```python
from build123d import *

# Parameters (mm, degrees)
SKETCH1_W               = 27
SKETCH1_H               = 22
SKETCH1_R               = 1.5
BOSS_EXTRUDE1_DEPTH     = 3
SKETCH2_W               = 3.5
SKETCH2_H               = 17
BOSS_EXTRUDE2_DEPTH     = 17
CUT_EXTRUDE1_DEPTH      = 28.451092874
CUT_EXTRUDE1_DEPTH_BACK = 28.451092874
SKETCH3_R               = 4
CUT_EXTRUDE2_DEPTH      = 28.451092874
CUT_EXTRUDE2_DEPTH_BACK = 28.451092874
SKETCH4_W               = 8.09758535
SKETCH4_H               = 1.5
FILLET1_R               = 3
FILLET2_R               = 3


with BuildPart() as part:
    # Sketch1 → Boss-Extrude1 (new body)
    with BuildSketch(Plane.XY):
        Rectangle(SKETCH1_W, SKETCH1_H)
        with Locations((10.5, 8.5)):
            Circle(SKETCH1_R, mode=Mode.SUBTRACT)
        with Locations((10.5, -8.5)):
            Circle(SKETCH1_R, mode=Mode.SUBTRACT)
        with Locations((-10.5, -8.5)):
            Circle(SKETCH1_R, mode=Mode.SUBTRACT)
        with Locations((-10.5, 8.5)):
            Circle(SKETCH1_R, mode=Mode.SUBTRACT)
    extrude(amount=BOSS_EXTRUDE1_DEPTH)

    # Sketch2 → Boss-Extrude2 (add)
    with BuildSketch(Plane.XY.offset(3)):
        Rectangle(SKETCH2_W, SKETCH2_H)
    extrude(amount=BOSS_EXTRUDE2_DEPTH)

    # Sketch3 → Cut-Extrude1 (cut, two sides: drawn at the far end of the back side and taken through both)
    with BuildSketch(Plane(origin=(1.75, 0, 0), x_dir=(0, 0, -1), z_dir=(1, 0, 0)).offset(-CUT_EXTRUDE1_DEPTH_BACK)):
        with Locations(Location((-13, 0, 0), (0, 0, 90))):
            Circle(SKETCH3_R)
    extrude(amount=CUT_EXTRUDE1_DEPTH + CUT_EXTRUDE1_DEPTH_BACK, mode=Mode.SUBTRACT)

    # Sketch4 → Cut-Extrude2 (cut, two sides: drawn at the far end of the back side and taken through both)
    with BuildSketch(Plane(origin=(1.75, 0, 0), x_dir=(0, 0, -1), z_dir=(1, 0, 0)).offset(-CUT_EXTRUDE2_DEPTH_BACK)):
        with Locations((-18.330812417, 0)):
            Rectangle(SKETCH4_W, SKETCH4_H)
    extrude(amount=CUT_EXTRUDE2_DEPTH + CUT_EXTRUDE2_DEPTH_BACK, mode=Mode.SUBTRACT)

    # Fillet1
    fillet1_edges = [part.edges().sort_by_distance(p)[0] for p in [
        (-1.75, 0, 3),
        (1.75, 0, 3),
    ]]
    fillet(fillet1_edges, radius=FILLET1_R)

    # Fillet2
    fillet2_edges = [part.edges().sort_by_distance(p)[0] for p in [
        (0, -8.5, 20),
        (0, 8.5, 20),
    ]]
    fillet(fillet2_edges, radius=FILLET2_R)


solid = part.part
```
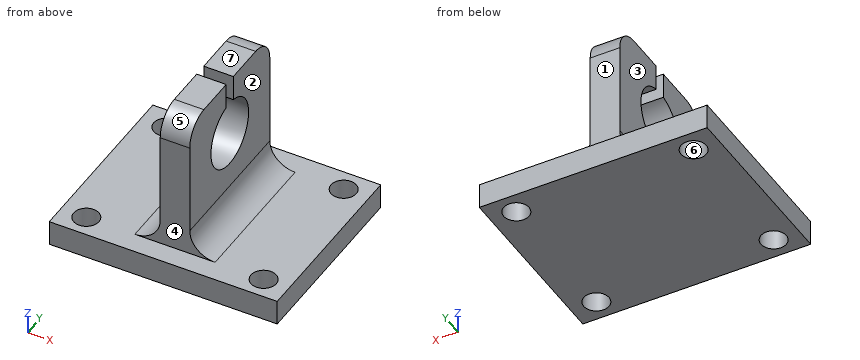
Could you check a few things on this model? Use its own coordinates, in mm. Face numbers are marked on the shaded views. A direction names the side the tool comes from. Round coordinates to 2 decimals unless told otherwise and drop trailing zeros. Loops run counter-clockwise (first coordinate to the right, second up) from the corner with the lowest first, then second, coordinate; pieces in that order, holes last. Notation, with made-up numbers: M 53.5,53 L 103.5,53 A35 ccw 103.5,91 Z; hole C 64.25,68.5 d9. An arc over 180 degrees is marked long. Write item = value, one per line.
1. Which directions (+Z, -Z, +X, -X, +Y, -Y) give clear straight access to the entire face, cutting with the end or side of a thin tool? Please do the marked faces 1, 2, 3 and 4.
Results below:
face_1 = +Z, +X, -X, +Y
face_2 = +Z, +X, +Y, -Y
face_3 = +Z, -X, +Y, -Y
face_4 = +Z, +X, -X, -Y
2. Will these pins go through, and if not, where does the flat tip stop? P1, Ø7, axis at y = 0, z = 13, coming from the -X side; P2, Ø7, axis at y = -1.5, z = 11.5, coming from the +X side; P3, Ø10, axis at x = -9.5, y = 5, coming from the +Z side; P4, Ø3, axis at x = -1.5, z = 9.5, coming from the +Y side.
Results below:
P1 = through
P2 = 1.75
P3 = 3.01
P4 = 8.5
3. I want a section at D-D, the plane y = 9. Write out the boundary of the cut face in (x, z), and give its area (3 significant figures).
Results below:
outline = M -13.5,0 L -11.91,0 L -11.91,3 L -13.5,3 Z; M -9.09,0 L 9.09,0 L 9.09,3 L -9.09,3 Z; M 11.91,0 L 13.5,0 L 13.5,3 L 11.91,3 Z
area = 64.0 mm²
4. I want a section at C-C, the plane y = 0. Write out the boundary of the cut face in (x, z), and give its area (3 significant figures).
Results below:
outline = M -13.5,0 L 13.5,0 L 13.5,3 L 4.75,3 A3 cw 1.75,6 L 1.75,9 L -1.75,9 L -1.75,6 A3 cw -4.75,3 L -13.5,3 Z
area = 106 mm²
5. Thinking about a two-plate mould opening in Y: for the marked faces 5, 6 and 7, which applies, +Y half, -Y half, draft (parallel to the pull), parting line (faces both ways), or undercut?
Results below:
face_5 = -Y half
face_6 = undercut
face_7 = draft
6. I want a section at A-A, the plane x = 10.5. Write out the boundary of the cut face in (y, z).
Results below:
outline = M -11,0 L -10,0 L -10,3 L -11,3 Z; M -7,0 L 7,0 L 7,3 L -7,3 Z; M 10,0 L 11,0 L 11,3 L 10,3 Z
7. I want a section at B-B, the plane z = 13. Write out the boundary of the cut face in (x, y).
Results below:
outline = M -1.75,-8.5 L 1.75,-8.5 L 1.75,-4 L -1.75,-4 Z; M -1.75,4 L 1.75,4 L 1.75,8.5 L -1.75,8.5 Z
8. I need wall thicknesses on probe 1 along Y at (x, z) = (10.5, 1.9); probe 2 along X at (y, z) = (5.25, 14); probe 3 along Z at (x, y) = (-6.75, 2). Which ranges of each line are inside material? Lowest first, please.
Results below:
probe_1 = -11 to -10, -7 to 7, 10 to 11
probe_2 = -1.75 to 1.75
probe_3 = 0 to 3
